Could you check a few things on this model? Use its own coordinates, in mm. Face numbers are marked on the shaded views. A direction names the side the tool comes from. Round coordinates to 2 decimals unless told otherwise and drop trailing zeros. Loops run counter-clockwise (first coordinate to the right, second up) from the corner with the lowest first, then second, coordinate; pieces in that order, holes last. Notation, with made-up numbers: (48, 63) -> (94, 63) arc R17 ccw to (94, 94) -> close; hole circle Ø9 at (58, 41.5). An arc over 180 degrees is marked (long way). One line per item, written item: value.
from build123d import *

# Parameters (mm, degrees)
SKETCH1_R                    = 1
EXTRUDE1_DEPTH               = 4
SKETCH1_3_R                  = 2.38125
EXTRUDE4_DEPTH               = 2
M2X0_4_TAPPED_HOLE1_D        = 1.6
M2X0_4_TAPPED_HOLE1_DEPTH    = 3
M2X0_4_TAPPED_HOLE1_TIP      = 0.480688495
F_2_0_2_DIAMETER_HOLE1_D     = 2
F_2_0_2_DIAMETER_HOLE1_DEPTH = 10
F_2_0_2_DIAMETER_HOLE1_TIP   = 0.600860619


with BuildPart() as part:
    # Sketch1 → Extrude1 (new body)
    with BuildSketch(Plane(origin=(0, 0, 0), x_dir=(1, 0, 0), z_dir=(0, 1, 0))):
        with BuildLine():
            Line((-5.186041147, 3.316192399), (2.637731834, -10.234979911))
            ThreePointArc((2.637731834, -10.234979911), (4.802795343, -11.484979911), (6.967858853, -10.234979911))
            Line((6.967858853, -10.234979911), (14.791631834, 3.316192399))
            ThreePointArc((14.791631834, 3.316192399), (14.791631834, 5.816192399), (12.626568324, 7.066192399))
            Line((12.626568324, 7.066192399), (-3.020977638, 7.066192399))
            ThreePointArc((-3.020977638, 7.066192399), (-5.186041147, 5.816192399), (-5.186041147, 3.316192399))
        make_face()
        with Locations((-2.110635714, 4.040606244)):
            Circle(SKETCH1_R, mode=Mode.SUBTRACT)
        with Locations((11.7162264, 4.040606244)):
            Circle(SKETCH1_R, mode=Mode.SUBTRACT)
        with Locations((4.802795343, -7.933807601)):
            Circle(SKETCH1_R, mode=Mode.SUBTRACT)
    extrude(amount=EXTRUDE1_DEPTH)

    # Sketch1_3 → Extrude4 (cut)
    with BuildSketch(Plane(origin=(0, 0, 0), x_dir=(1, 0, 0), z_dir=(0, 1, 0))):
        with Locations((4.802795343, -7.933807601)):
            Circle(SKETCH1_3_R)
        with Locations((11.7162264, 4.040606244)):
            Circle(SKETCH1_3_R)
        with Locations((-2.110635714, 4.040606244)):
            Circle(SKETCH1_3_R)
    extrude(amount=EXTRUDE4_DEPTH, mode=Mode.SUBTRACT)

    # M2x0.4 Tapped Hole1
    with Locations(Plane(origin=(4.802795343, 0, -0.049134963), x_dir=(0, 0, -1), z_dir=(0, -1, 0))):
        with Locations((0, 0)):
            Hole(M2X0_4_TAPPED_HOLE1_D / 2, depth=M2X0_4_TAPPED_HOLE1_DEPTH)
            with Locations((0, 0, -(M2X0_4_TAPPED_HOLE1_DEPTH + M2X0_4_TAPPED_HOLE1_TIP / 2))):  # 118° drill point
                Cone(0, M2X0_4_TAPPED_HOLE1_D / 2, M2X0_4_TAPPED_HOLE1_TIP, mode=Mode.SUBTRACT)

    # 2.0 _2_ Diameter Hole1
    with Locations(Plane(origin=(0.457896151, 0, 2.459393756), x_dir=(0, 0, -1), z_dir=(0, -1, 0))):
        with Locations((0, 0), (0, 8.689798385), (7.525586155, 4.344899192)):
            Hole(F_2_0_2_DIAMETER_HOLE1_D / 2, depth=F_2_0_2_DIAMETER_HOLE1_DEPTH)
            with Locations((0, 0, -(F_2_0_2_DIAMETER_HOLE1_DEPTH + F_2_0_2_DIAMETER_HOLE1_TIP / 2))):  # 118° drill point
                Cone(0, F_2_0_2_DIAMETER_HOLE1_D / 2, F_2_0_2_DIAMETER_HOLE1_TIP, mode=Mode.SUBTRACT)


solid = part.part
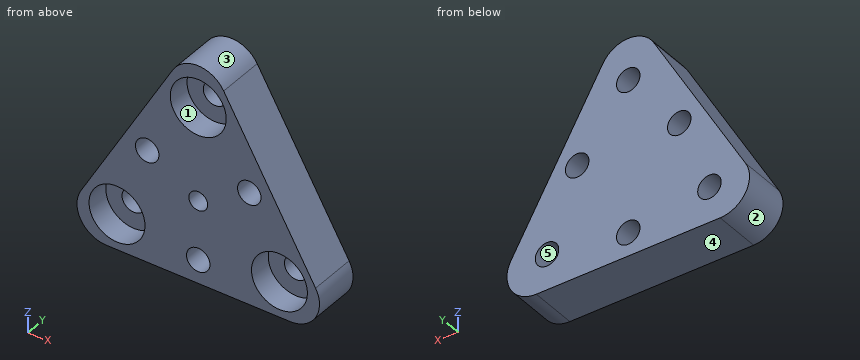
(1) If we section it at A-A, the plane x = -2: Please give me the cut outline in (y, z).
Recorded:
outline: (0, -7.07) -> (4, -7.07) -> (4, -5.03) -> (2, -5.03) -> (2, -6.42) -> (0, -6.42) -> close; (0, -1.66) -> (2, -1.66) -> (2, -3.05) -> (4, -3.05) -> (4, 2.2) -> (0, 2.2) -> close
(2) If we section it at B-B, the plane y = 2.6: Please give me the cut outline in (x, z), then the cut area to 3 significant figures.
Recorded:
outline: (-5.19, -3.32) arc R2.5 ccw to (-3.02, -7.07) -> (12.63, -7.07) arc R2.5 ccw to (14.79, -3.32) -> (6.97, 10.23) arc R2.5 ccw to (2.64, 10.23) -> close; hole circle Ø2 at (-2.11, -4.04); hole circle Ø2 at (0.46, 2.46); hole circle Ø2 at (4.8, -5.07); hole circle Ø2 at (4.8, 7.93); hole circle Ø1.6 at (4.8, -0.05); hole circle Ø2 at (9.15, 2.46); hole circle Ø2 at (11.72, -4.04)
area: 222 mm²
(3) If I drill on L1, parallel to Z at x = 4.75, y = 1.75; L2, parallel to X at y = 0.3, z = -3.25; L3, parallel to X at y = 2.1, z = 2.5, over which ranges is the centre line in solid material (lowest first)?
Recorded:
L1: -7.07 to -6.06, -4.07 to -0.85, 0.75 to 5.55, 10.31 to 11.48
L2: -5.15 to -4.36, 0.14 to 9.47, 13.96 to 14.75
L3: -1.83 to -0.54, 1.46 to 8.15, 10.15 to 11.43
(4) If we section it at C-C, the plane z = 6.5: Please give me the cut outline in (x, y), then the cut area to 3 significant figures.
Recorded:
outline: (0.48, 0) -> (2.9, 0) -> (2.9, 2) -> (6.7, 2) -> (6.7, 0) -> (9.12, 0) -> (9.12, 4) -> (0.48, 4) -> close
area: 27.0 mm²
(5) I'm going to push flat-ended pins straight in: pin 1 Ø4.5 at (x, z) = (11.72, -4.04) entering from -Y; pin 2 Ø1.6 at (x, z) = (-2.11, -4.04) entering from +Y; pin 3 Ø2 at (x, y) = (9.5, 2.5) entering from +Z; pin 4 Ø1.5 at (y, z) = (0.5, 8.5) entering from -X. Where does each tip first touch, or does it pass through?
Recorded:
pin 1: y = 2
pin 2: through
pin 3: z = 7.58
pin 4: x = 1.2
(6) For the marked faces 1 and 2, which set-ups out of +Z, -Z, +X, -X, +Y, -Y let a thin tool reach every point of the face, with its end or its side?
Recorded:
face 1: -Y
face 2: -X, +Y, -Y
(7) Thinking about a two-plate mould opening in X: for the marked faces 3, 4 and 5, which applies, released by +X, released by -X, zero draft, split by the parting line, or undercut?
Recorded:
face 3: split by the parting line
face 4: zero draft
face 5: undercut
(8) If we section it at D-D, the plane x = 3: Please give me the cut outline in (y, z), then the cut area to 3 significant figures.
Recorded:
outline: (0, -7.07) -> (4, -7.07) -> (4, 10.72) -> (0, 10.72) -> (0, 9.49) -> (2, 9.49) -> (2, 6.38) -> (0, 6.38) -> close
area: 64.9 mm²
